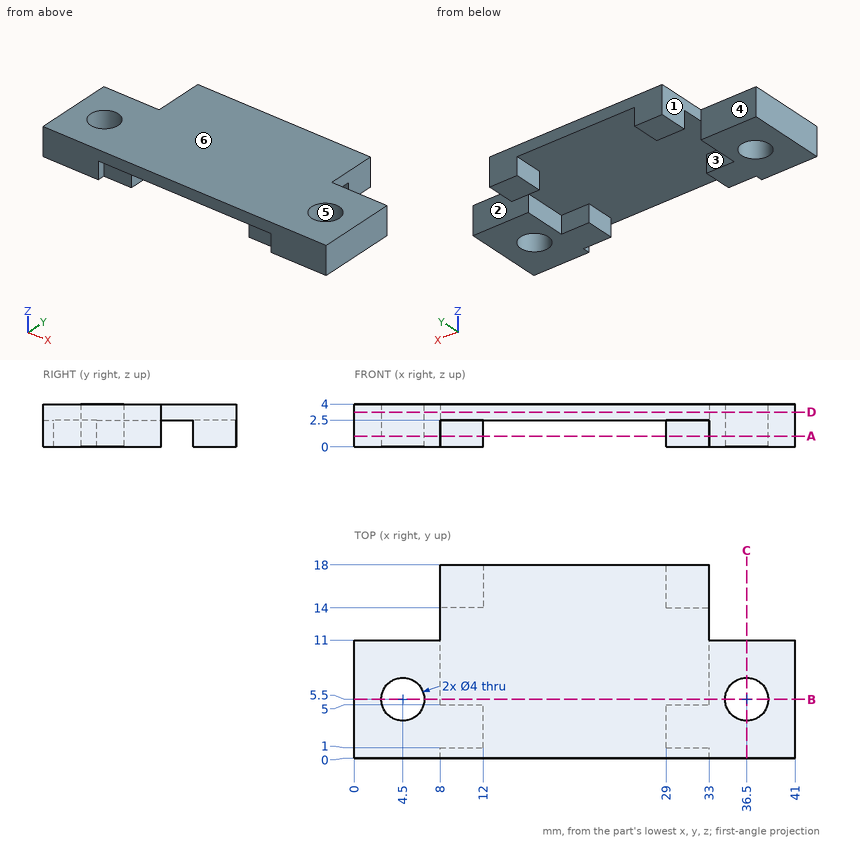
The figure shows three views and two pictorial views of one solid part (mm, origin at its lowest corner). Answer the questions. A direction names the side the tool comes from. Round coordinates to 2 decimals unless told otherwise and drop trailing zeros. Order: outer loops, then holes, each group sorted by start corner. A loop starts at its lowest first (then second) coordinate and runs counter-clockwise, first axis right, second up. Notation, with made-up numbers: M -37.75,87.25 L 10.25,87.25 A27 ccw 10.25,107.25 Z; hole C 60,75 d9. An arc over 180 degrees is marked long. Put each result on its own line as item: value. Start each with the question number.
Q1. For a pull along Y with two mould halves and no side action, classify the marked faces 4, 5 and 6 as pulls with the +Y half, pulls with the -Y half, needs draft (parallel to the pull), parting line crosses it, or undercut.
Q2. Section A-A, the plane z = 1 is taken. Write down the section's boundary in (x, y), and give its area (3 significant figures).
Q3. Straight lines are drawn through the part: L1, parallel to X at y = 5.5, z = 1.85; L2, parallel to X at y = 5.5, z = 2.7; L3, parallel to X at y = 3.25, z = 2.3. For each, find the intervals that lie inside material, in ascending order. Write a range as [from, to].
Q4. Section D-D, the plane z = 3.25 is taken. Write down the section's boundary in (x, y).
Q5. A tool of negligible diameter and unlimited length cuts with its end or side. For the marked faces 1, 2 and 3, from which of +Z, -Z, +X, -X, +Y, -Y can it reach the whole face along a straight path? Write none if from no direction.
Q6. Section B-B, the plane y = 5.5 is taken. Write down the section's boundary in (x, z).
Q7. Flat-ended cylindrical pins translate along their axes: pin 1 (1.2 mm diameter, centred on y = 17, z = 1.5, fed in from -X); pin 2 (1 mm diameter, centred on x = 24.5, z = 0.5, fed in from -Y). Find the tip coordinate at first contact, or state that the pin passes through.
Q8. Section C-C, the plane x = 36.5 is taken. Write down the section's boundary in (y, z), and give its area (3 significant figures).
Findings below:
1. face 4: pulls with the +Y half
1. face 5: undercut
1. face 6: needs draft
2. outline: M 0,0 L 8,0 L 8,1 L 12,1 L 12,5 L 8,5 L 8,11 L 0,11 Z; M 8,14 L 12,14 L 12,18 L 8,18 Z; M 29,1 L 33,1 L 33,0 L 41,0 L 41,11 L 33,11 L 33,5 L 29,5 Z; M 29,14 L 33,14 L 33,18 L 29,18 Z; hole C 4.5,5.5 d4; hole C 36.5,5.5 d4
2. area: 215 mm^2
3. L1: x = [0, 2.5], [6.5, 8], [33, 34.5], [38.5, 41]
3. L2: x = [0, 2.5], [6.5, 34.5], [38.5, 41]
3. L3: x = [0, 12], [29, 41]
4. outline: M 0,0 L 41,0 L 41,11 L 33,11 L 33,18 L 8,18 L 8,11 L 0,11 Z; hole C 4.5,5.5 d4; hole C 36.5,5.5 d4
5. face 1: +Z, -Z, -X, +Y
5. face 2: +Z, -Z, +X, +Y
5. face 3: -Z
6. outline: M 0,0 L 2.5,0 L 2.5,4 L 0,4 Z; M 6.5,0 L 8,0 L 8,2.5 L 33,2.5 L 33,0 L 34.5,0 L 34.5,4 L 6.5,4 Z; M 38.5,0 L 41,0 L 41,4 L 38.5,4 Z
7. pin 1: stops at x = 8
7. pin 2: passes through
8. outline: M 0,0 L 3.5,0 L 3.5,4 L 0,4 Z; M 7.5,0 L 11,0 L 11,4 L 7.5,4 Z
8. area: 28.0 mm^2
